Design review of the part built by this model. Coordinates are the model's own, in mm. A direction names the side the tool comes from. Give positions to 0.01 mm unless a question says otherwise; leave off trailing zeros. Order: outer loops, then holes, each group sorted by start corner. A loop starts at its lowest first (then second) coordinate and runs counter-clockwise, first axis right, second up. Notation, with made-up numbers: M -26.5,77 L -0.5,77 A25 cw -0.5,95 Z; hole C 76,-1 d6. An arc over 180 degrees is marked long. Put each result on its own line as item: value. Start each with the question number.
from build123d import *

# Parameters (mm, degrees)
BOSS_EXTRUDE1_DEPTH     = 1
BOSS_EXTRUDE2_DEPTH     = 2
SKETCH3_R               = 1.55
CUT_EXTRUDE1_DEPTH      = 22.313141486
CUT_EXTRUDE2_DEPTH      = 2
CUT_EXTRUDE2_DEPTH_BACK = 1.7
SKETCH4_R               = 2.85
CUT_EXTRUDE3_DEPTH      = 2
SKETCH6_R               = 2.875
CUT_EXTRUDE4_DEPTH      = 22.195518394
CHAMFER1_SIZE           = 0.1
SKETCH7_R               = 4
CUT_EXTRUDE5_DEPTH      = 0.3


with BuildPart() as part:
    # Sketch1 → Boss-Extrude1 (new body)
    with BuildSketch(Plane(origin=(0, 0, 0), x_dir=(1, 0, 0), z_dir=(0, 1, 0))):
        with BuildLine():
            Line((14.823825022, -5), (-14.823825022, -5))
            ThreePointArc((-14.823825022, -5), (-14.997328014, -4.984833342), (-15.165568085, -4.939793423))
            Line((-15.165568085, -4.939793423), (-19.841743063, -3.239366159))
            ThreePointArc((-19.841743063, -3.239366159), (-20.319067477, -2.873269928), (-20.5, -2.299572735))
            Line((-20.5, -2.299572735), (-20.5, 2.299572735))
            ThreePointArc((-20.5, 2.299572735), (-20.319067477, 2.873269928), (-19.841743063, 3.239366159))
            Line((-19.841743063, 3.239366159), (-15.165568085, 4.939793423))
            ThreePointArc((-15.165568085, 4.939793423), (-14.997328014, 4.984833342), (-14.823825022, 5))
            Line((-14.823825022, 5), (14.823825022, 5))
            ThreePointArc((14.823825022, 5), (14.997328014, 4.984833342), (15.165568085, 4.939793423))
            Line((15.165568085, 4.939793423), (19.841743063, 3.239366159))
            ThreePointArc((19.841743063, 3.239366159), (20.319067477, 2.873269928), (20.5, 2.299572735))
            Line((20.5, 2.299572735), (20.5, -2.299572735))
            ThreePointArc((20.5, -2.299572735), (20.319067477, -2.873269928), (19.841743063, -3.239366159))
            Line((19.841743063, -3.239366159), (15.165568085, -4.939793423))
            ThreePointArc((15.165568085, -4.939793423), (14.997328014, -4.984833342), (14.823825022, -5))
        make_face()
    extrude(amount=BOSS_EXTRUDE1_DEPTH)

    # Sketch2 → Boss-Extrude2 (add)
    with BuildSketch(Plane(origin=(0, 1, 0), x_dir=(1, 0, 0), z_dir=(0, 1, 0))):
        with BuildLine():
            Line((11.332922852, -5), (-11.332922852, -5))
            ThreePointArc((-11.332922852, -5), (-11.497715753, -4.986328191), (-11.65800262, -4.945686599))
            Line((-11.65800262, -4.945686599), (-18.825079769, -2.48200383))
            ThreePointArc((-18.825079769, -2.48200383), (-19.31396553, -2.117230404), (-19.5, -1.53631723))
            Line((-19.5, -1.53631723), (-19.5, 1.53631723))
            ThreePointArc((-19.5, 1.53631723), (-19.31396553, 2.117230404), (-18.825079769, 2.48200383))
            Line((-18.825079769, 2.48200383), (-11.65800262, 4.945686599))
            ThreePointArc((-11.65800262, 4.945686599), (-11.497715753, 4.986328191), (-11.332922852, 5))
            Line((-11.332922852, 5), (11.332922852, 5))
            ThreePointArc((11.332922852, 5), (11.497715753, 4.986328191), (11.65800262, 4.945686599))
            Line((11.65800262, 4.945686599), (18.825079769, 2.48200383))
            ThreePointArc((18.825079769, 2.48200383), (19.31396553, 2.117230404), (19.5, 1.53631723))
            Line((19.5, 1.53631723), (19.5, -1.53631723))
            ThreePointArc((19.5, -1.53631723), (19.31396553, -2.117230404), (18.825079769, -2.48200383))
            Line((18.825079769, -2.48200383), (11.65800262, -4.945686599))
            ThreePointArc((11.65800262, -4.945686599), (11.497715753, -4.986328191), (11.332922852, -5))
        make_face()
    extrude(amount=BOSS_EXTRUDE2_DEPTH)

    # Sketch3 → Cut-Extrude1 (cut, through all)
    with BuildSketch(Plane(origin=(0, 3, 0), x_dir=(1, 0, 0), z_dir=(0, 1, 0))):
        with Locations(Location((-16, 0, 0), (0, 0, 270))):
            Circle(SKETCH3_R)
        with Locations(Location((16, 0, 0), (0, 0, 270))):
            Circle(SKETCH3_R)
    extrude(amount=-CUT_EXTRUDE1_DEPTH, mode=Mode.SUBTRACT)

    # Sketch4 → Cut-Extrude2 (cut, two sides: drawn at the far end of the back side and taken through both)
    with BuildSketch(Plane(origin=(0, 3, 0), x_dir=(1, 0, 0), z_dir=(0, 1, 0)).offset(-CUT_EXTRUDE2_DEPTH_BACK)):
        with Locations(Location((-16, 0, 0), (0, 0, 270))):
            Circle(SKETCH4_R)
        with Locations(Location((16, 0, 0), (0, 0, 270))):
            Circle(SKETCH4_R)
    extrude(amount=CUT_EXTRUDE2_DEPTH + CUT_EXTRUDE2_DEPTH_BACK, mode=Mode.SUBTRACT)

    # Sketch5 → Cut-Extrude3 (cut)
    with BuildSketch(Plane(origin=(0, 3, 0), x_dir=(1, 0, 0), z_dir=(0, 1, 0))):
        with BuildLine():
            Line((8.589484596, -4), (-8.589484596, -4))
            ThreePointArc((-8.589484596, -4), (-8.991616341, -3.959155446), (-9.377323193, -3.83829006))
            Line((-9.377323193, -3.83829006), (-11.287838597, -3.019497744))
            ThreePointArc((-11.287838597, -3.019497744), (-12.169682184, -2.282189702), (-12.5, -1.181207684))
            Line((-12.5, -1.181207684), (-12.5, 1.181207684))
            ThreePointArc((-12.5, 1.181207684), (-12.169682184, 2.282189702), (-11.287838597, 3.019497744))
            Line((-11.287838597, 3.019497744), (-9.377323193, 3.83829006))
            ThreePointArc((-9.377323193, 3.83829006), (-8.991616341, 3.959155446), (-8.589484596, 4))
            Line((-8.589484596, 4), (8.589484596, 4))
            ThreePointArc((8.589484596, 4), (8.991616341, 3.959155446), (9.377323193, 3.83829006))
            Line((9.377323193, 3.83829006), (11.287838597, 3.019497744))
            ThreePointArc((11.287838597, 3.019497744), (12.169682184, 2.282189702), (12.5, 1.181207684))
            Line((12.5, 1.181207684), (12.5, -1.181207684))
            ThreePointArc((12.5, -1.181207684), (12.169682184, -2.282189702), (11.287838597, -3.019497744))
            Line((11.287838597, -3.019497744), (9.377323193, -3.83829006))
            ThreePointArc((9.377323193, -3.83829006), (8.991616341, -3.959155446), (8.589484596, -4))
        make_face()
    extrude(amount=-CUT_EXTRUDE3_DEPTH, mode=Mode.SUBTRACT)

    # Sketch6 → Cut-Extrude4 (cut, through all)
    with BuildSketch(Plane(origin=(0, 1, 0), x_dir=(1, 0, 0), z_dir=(0, 1, 0))):
        with Locations(Location((-6.025, 0, 0), (0, 0, 270))):
            Circle(SKETCH6_R)
        with Locations(Location((6.025, 0, 0), (0, 0, 270))):
            Circle(SKETCH6_R)
    extrude(amount=-CUT_EXTRUDE4_DEPTH, mode=Mode.SUBTRACT)

    # Chamfer1
    chamfer1_edges = [part.edges().sort_by_distance(p)[0] for p in [
        (-19.31396553, 3, -2.117230404),
        (-19.5, 3, 0),
        (-19.31396553, 3, 2.117230404),
        (-15.241541194, 3, 3.713845214),
        (-11.497715753, 3, 4.986328191),
        (0, 3, 5),
        (11.497715753, 3, 4.986328191),
        (15.241541194, 3, 3.713845214),
        (19.31396553, 3, 2.117230404),
        (19.5, 3, 0),
        (19.31396553, 3, -2.117230404),
        (15.241541194, 3, -3.713845214),
        (11.497715753, 3, -4.986328191),
        (0, 3, -5),
        (-11.497715753, 3, -4.986328191),
        (-15.241541194, 3, -3.713845214),
    ]]
    chamfer(chamfer1_edges, length=CHAMFER1_SIZE)

    # Sketch7 → Cut-Extrude5 (cut)
    with BuildSketch(Plane.XZ):
        with Locations(Location((-16, 0, 0), (0, 0, 270))):
            Circle(SKETCH7_R)
        with Locations(Location((16, 0, 0), (0, 0, 270))):
            Circle(SKETCH7_R)
    extrude(amount=-CUT_EXTRUDE5_DEPTH, mode=Mode.SUBTRACT)


solid = part.part
1. Consider section C-C on x = -2.5. Give the boundary of the cut face in (y, z), then the cut area to 3 significant figures.
2. Consider section B-B on y = 2.15. Give the number of separate pieces and of enclosed holes in the cut face, then the cut area to 3 significant figures.
3. Machinability: for faces 4 (the cylindrical face through (-19.32, 1.94, -2.11)), 5 (the flat face through (12.5, 2, 0)), 6 (the flat face through (14, 0.3, 0)), which of the approach directions +Z, -Z, +X, -X, +Y, -Y give a long, thin tool a straight path to every point of the face, cutting with its end or side? Answer none if there is none.
4. Insertion check: pin 1 (4.5 mm diameter, centred on x = 16, z = -1, fed in from +Y); pin 2 (5 mm diameter, centred on x = -16, z = 0, fed in from -Y); pin 3 (1.5 mm diameter, centred on y = 2.5, z = 0, fed in from +X); pin 4 (3 mm diameter, centred on x = -15.5, z = 0.5, fed in from +Y). Each pin has a flat end and moves straight along its axis. Give the tip position at first contact, or say it passes through.
5. To check wall thickness, follow probe 1 along X at (y, z) = (0.65, 0); probe 2 along X at (y, z) = (1.55, 0.5); probe 3 along Z at (x, y) = (-11, 1.55). State the ranges of each line that lie inside material, in increasing order.
6. The part is to be moulded in two halves that separate along X. For faces 1 (the cylindrical face through (-8.832, 0.507, -0.623)), 2 (the cylindrical face through (20.3, 0.5, 2.9)), 3 (the flat face through (1.5, 3, -4.4)), say which applies: +X half, -X half, draft (parallel to the pull), parting line (faces both ways), or undercut.
7. Consider section A-A on x = 3.5. Give the boundary of the cut face in (y, z).
Returned:
1. outline: M 0,-5 L 2.9,-5 L 3,-4.9 L 3,-4 L 1,-4 L 1,4 L 3,4 L 3,4.9 L 2.9,5 L 0,5 Z
1. area: 14.0 mm2
2. separate pieces: 1
2. enclosed holes: 3
2. area: 106 mm2
3. face 4: -Z, -X, +Y
3. face 5: +Y
3. face 6: -Y
4. pin 1: stops at y = 3
4. pin 2: stops at y = 0.3
4. pin 3: stops at x = 19.5
4. pin 4: stops at y = 1.3
5. probe 1: x = -20.5 to -17.55, -14.45 to -8.9, -3.15 to 3.15, 8.9 to 14.45, 17.55 to 20.5
5. probe 2: x = -19.5 to -18.81, -13.19 to -12.5, 12.5 to 13.19, 18.81 to 19.5
5. probe 3: z = -5 to -3.14, 3.14 to 5
6. face 1: undercut
6. face 2: +X half
6. face 3: draft
7. outline: M 0,-5 L 2.9,-5 L 3,-4.9 L 3,-4 L 1,-4 L 1,-1.37 L 0,-1.37 Z; M 0,1.37 L 1,1.37 L 1,4 L 3,4 L 3,4.9 L 2.9,5 L 0,5 Z
